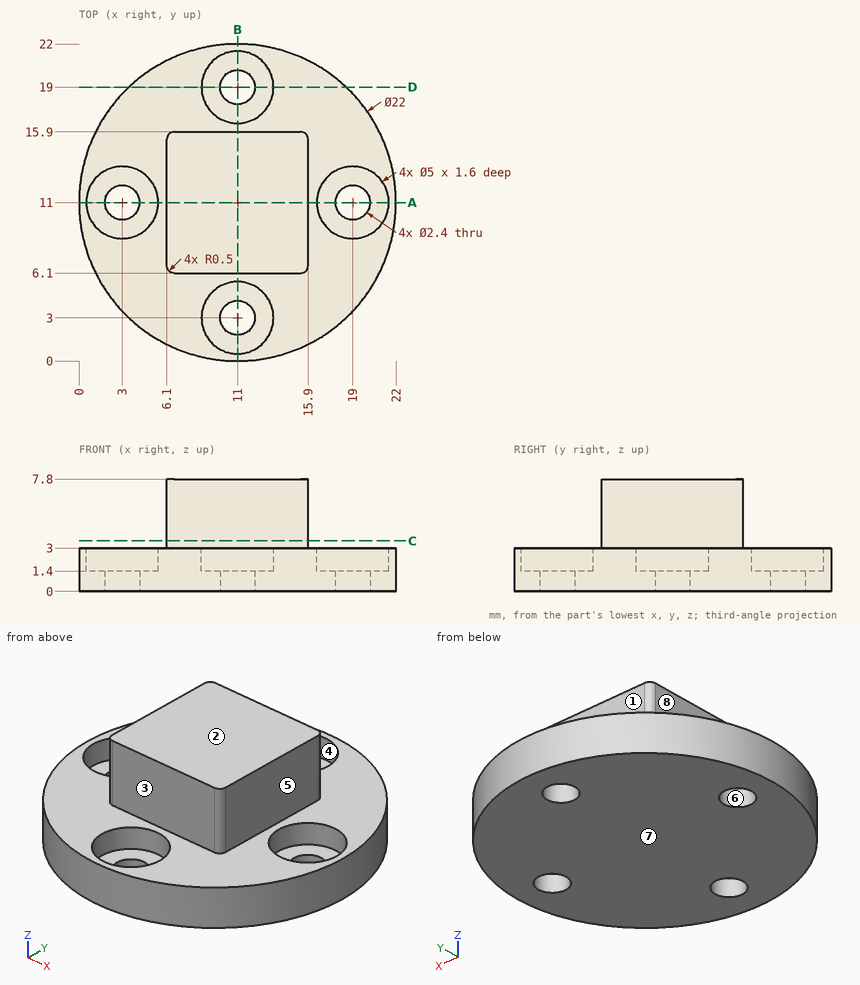
Geometry: see drawing. Coordinates: mm, zero at the bounding-box minimum. A direction names the side the tool comes from. Give positions to 0.01 mm unless a question says otherwise; leave off trailing zeros. Loops run counter-clockwise (first coordinate to the right, second up) from the corner with the lowest first, then second, coordinate; pieces in that order, holes last. Notation, with made-up numbers: (57.25, 18) - (106.25, 18) arc R17 ccw to (106.25, 25) - close; hole circle Ø6 at (-20.75, 45). An arc over 180 degrees is marked (long way). Answer as CSV lines item,"result". Start each with the question number.
1. Section D-D, the plane y = 19. Return loops of the section in (x, z), plus the area to 3 significant figures.
2. Section C-C, the plane z = 3.5. Return loops of the section in (x, y), plus the area to 3 significant figures.
3. Reachability of the marked faces 1, 2, 3, 4 and 5 from +Z, -Z, +X, -X, +Y, -Y: full face, straight path, thin tool, end or side. Return the list, or none.
4. Section A-A, the plane y = 11. Return loops of the section in (x, z), plus the area to 3 significant figures.
5. Ray query, L1, parallel to Y at x = 11, z = 1.9; L2, parallel to Y at x = 10.5, z = 1.75; L3, parallel to Z at x = 18.25, y = 17.25. Return the intervals inside material, ascending.
6. Draft query along X for the marked faces 6, 7 and 8. Return one class per face: released by +X, released by -X, zero draft, split by the parting line, or undercut.
7. Pin query (flat end, axial travel): P1, Ø4, axis at x = 11, y = 6.5, coming from the -Z side; P2, Ø2.5, axis at y = 9.5, z = 6, coming from the -X side; P3, Ø5.5, axis at x = 19, y = 11, coming from the +Z side; P4, Ø2.5, axis at x = 3, y = 11, coming from the +Z side. Return the tip coordinate at first contact, or that it passes through.
Answers:
1,outline,"(3.45, 0) - (9.8, 0) - (9.8, 1.4) - (8.5, 1.4) - (8.5, 3) - (3.45, 3) - close; (12.2, 0) - (18.55, 0) - (18.55, 3) - (13.5, 3) - (13.5, 1.4) - (12.2, 1.4) - close"
1,area,"33.9 mm2"
2,outline,"(6.1, 6.6) arc R0.5 ccw to (6.6, 6.1) - (15.4, 6.1) arc R0.5 ccw to (15.9, 6.6) - (15.9, 15.4) arc R0.5 ccw to (15.4, 15.9) - (6.6, 15.9) arc R0.5 ccw to (6.1, 15.4) - close"
2,area,"95.8 mm2"
3,face 1,"+Z, +X, -X, +Y"
3,face 2,"+Z, +X, -X, +Y, -Y"
3,face 3,"+Z, +X, -X, -Y"
3,face 4,"+Z"
3,face 5,"+Z, +X, +Y, -Y"
4,outline,"(0, 0) - (1.8, 0) - (1.8, 1.4) - (0.5, 1.4) - (0.5, 3) - (0, 3) - close; (4.2, 0) - (17.8, 0) - (17.8, 1.4) - (16.5, 1.4) - (16.5, 3) - (15.9, 3) - (15.9, 7.8) - (6.1, 7.8) - (6.1, 3) - (5.5, 3) - (5.5, 1.4) - (4.2, 1.4) - close; (20.2, 0) - (22, 0) - (22, 3) - (21.5, 3) - (21.5, 1.4) - (20.2, 1.4) - close"
4,area,"90.3 mm2"
5,L1,"y = 0 to 0.5, 5.5 to 16.5, 21.5 to 22"
5,L2,"y = 0.01 to 0.55, 5.45 to 16.55, 21.45 to 21.99"
5,L3,"z = 0 to 3"
6,face 6,"undercut"
6,face 7,"zero draft"
6,face 8,"released by -X"
7,P1,"stops at z = 0"
7,P2,"stops at x = 6.1"
7,P3,"stops at z = 3"
7,P4,"stops at z = 1.4"
